Could you check a few things on this model? Use its own coordinates, in mm. A direction names the side the tool comes from. Give positions to 0.01 mm unless a question says otherwise; leave off trailing zeros. Loops run counter-clockwise (first coordinate to the right, second up) from the corner with the lowest first, then second, coordinate; pieces in that order, holes last. Notation, with made-up numbers: (-10.75, -2.75) -> (-3.75, -2.75) arc R17 ccw to (-3.75, 4.25) -> close; hole circle Ø8 at (56.25, 11.5). An arc over 180 degrees is marked (long way). Write each question's results on one line, items separated by ' | '. Start each with the question number.
Q1. We'd pull the mould along X, two halves only. Please class faces 1 (the face through (2.561, 0.2, -3.3)), 2 (the face through (-6.17, 1.48, 64.55)), 3 (the face through (-23, 3, 11)), 4 (the face through (-23.473, 1.479, 71.994)): released by +X, released by -X, zero draft, split by the parting line, or undercut.
Q2. Which directions (+Z, -Z, +X, -X, +Y, -Y) give clear straight access to the entire face, cutting with the end or side of a thin tool? Please do faces 5 (the face through (-23, -12, -55.512)), 6 (the face through (-23, 0, 13)).
Q3. If I drill on line 1 along Z through (x, y) = (-26, -23.5); line 2 along Y through (x, z) = (-33.5, 31.5), over which ranges is the centre line in solid material (lowest first)?
Q4. If we section it at B-B, the plane y = -24: List the corners of the cut face in (x, z) for me, plus the area to 3 significant figures.
Q5. Will these pins go through, and if not, where does the flat tip stop? P1, Ø1.5, axis at x = -26.5, z = 24.5, coming from the -Y side; P2, Ø6, axis at x = -4, y = -5.5, coming from the +Z side; P3, Ø10, axis at y = -9, z = 53, coming from the -X side.
Q6. If we section it at C-C, the plane z = -40.5: List the corners of the cut face in (x, y) for me.
Q7. If we section it at A-A, the plane x = -9: List the corners of the cut face in (y, z) for me, plus the area to 3 significant figures.
from build123d import *

# Parameters (mm, degrees)
SKETCH1_W           = 50
SKETCH1_H           = 135
BOSS_EXTRUDE1_DEPTH = 3
SKETCH2_W           = 50
SKETCH2_H           = 3
BOSS_EXTRUDE2_DEPTH = 28
SKETCH3_R           = 2.7
CUT_EXTRUDE1_DEPTH  = 90
SKETCH5_R           = 2.85
CUT_EXTRUDE2_DEPTH  = 90


with BuildPart() as part:
    # Sketch1 → Boss-Extrude1 (new body)
    with BuildSketch(Plane(origin=(0, 0, 0), x_dir=(1, 0, 0), z_dir=(0, 1, 0))):
        with Locations((-22.439180538, -11.987836108)):
            Rectangle(SKETCH1_W, SKETCH1_H)
    extrude(amount=BOSS_EXTRUDE1_DEPTH)

    # Sketch2 → Boss-Extrude2 (add)
    with BuildSketch(Plane.XZ):
        with Locations((-22.439180538, -54.012163892)):
            Rectangle(SKETCH2_W, SKETCH2_H)
    extrude(amount=BOSS_EXTRUDE2_DEPTH)

    # Sketch3 → Cut-Extrude1 (cut)
    with BuildSketch(Plane.XZ):
        with Locations(Location((-22.439180538, 74.487836108, 0), (0, 0, 270))):
            Circle(SKETCH3_R)
    extrude(amount=-CUT_EXTRUDE1_DEPTH, mode=Mode.SUBTRACT)

    # Sketch5 → Cut-Extrude2 (cut)
    with BuildSketch(Plane.XZ):
        with Locations(Location((-40.439180538, 62.287836108, 0), (0, 0, 270))):
            Circle(SKETCH5_R)
        with Locations(Location((-4.439180538, 62.287836108, 0), (0, 0, 270))):
            Circle(SKETCH5_R)
    extrude(amount=-CUT_EXTRUDE2_DEPTH, mode=Mode.SUBTRACT)


solid = part.part
Final values:
1) face 1: released by +X | face 2: undercut | face 3: zero draft | face 4: undercut
2) face 5: -Z, +X, -X, +Y, -Y | face 6: +Z, +X, -X, -Y
3) line 1: z = -55.51 to -52.51 | line 2: y = 0 to 3
4) outline: (-47.44, -55.51) -> (2.56, -55.51) -> (2.56, -52.51) -> (-47.44, -52.51) -> close | area: 150 mm²
5) P1: stops at y = 0 | P2: stops at z = -52.51 | P3: passes through
6) outline: (-47.44, 0) -> (2.56, 0) -> (2.56, 3) -> (-47.44, 3) -> close
7) outline: (-28, -55.51) -> (3, -55.51) -> (3, 79.49) -> (0, 79.49) -> (0, -52.51) -> (-28, -52.51) -> close | area: 489 mm²
